Read the model definition and answer for the solid it produces. Units are mm, in the model's axes. A direction names the side the tool comes from. Give positions to 0.01 mm unless a question says otherwise; leave off trailing zeros. Loops run counter-clockwise (first coordinate to the right, second up) from the corner with the lowest first, then second, coordinate; pieces in that order, holes last. Notation, with made-up numbers: (49.5, -28) -> (79.5, -28) arc R23 cw to (79.5, -7) -> close; hole circle Ø3 at (63, 30). An arc over 180 degrees is marked (long way). Return JSON: item names as keys, results as strings. Group by question number.
from build123d import *

# Parameters (mm, degrees)
F0_W     = 76.2
F0_H     = 76.2
F1_DEPTH = 76.2
F2_W     = 58.42
F2_H     = 58.42
F3_DEPTH = 76.2
F4_W     = 58.42
F4_H     = 67.31
F5_DEPTH = 76.2
F6_W     = 58.42
F6_H     = 134.62
F7_DEPTH = 76.2


with BuildPart() as f1:
    # F0 (on Top) → F1 (new body)
    with BuildSketch(Plane.XY):
        with Locations((38.1, -38.1)):
            Rectangle(F0_W, F0_H)
    extrude(amount=F1_DEPTH)

    # F2 (on face) → F3 (cut)
    with BuildSketch(Plane.XY.offset(76.2)):
        with Locations((38.1, -38.1)):
            Rectangle(F2_W, F2_H)
    extrude(amount=-F3_DEPTH, mode=Mode.SUBTRACT)

    # F4 (on face) → F5 (cut)
    with BuildSketch(Plane.YZ.offset(76.2)):
        with Locations((-38.1, 33.655)):
            Rectangle(F4_W, F4_H)
    extrude(amount=-F5_DEPTH, mode=Mode.SUBTRACT)

    # F6 (on face) → F7 (cut)
    with BuildSketch(Plane.XZ.offset(76.2)):
        with Locations((38.1, 0)):
            Rectangle(F6_W, F6_H)
    extrude(amount=-F7_DEPTH, mode=Mode.SUBTRACT)


solid = f1.part
1. Which of the six approach directions +Z, -Z, +X, -X, +Y, -Y give full straight-line access (tool end or side, diameter ignored) to faces 5 (the flat face through (72, -39, 67.31)), 6 (the flat face through (38, -76.2, 69)), 7 (the flat face through (8.89, -72, 33)), 8 (the flat face through (4, -72, 0)), 9 (the flat face through (67.31, -39, 72))?
2. Section B-B on z = 33.5 is taken. Determine the outline of the cut face in (x, y), then the cut area to 3 significant figures.
3. A flat-ended cylindrical pin translates along its axis: pin 1 Ø4.5 at (x, y) = (72.5, -27.5) entering from -Z. Find the tip coordinate at first contact, or state that the pin passes through.
4. Section D-D on z = 71.5 is taken. Determine the outline of the cut face in (x, y).
5. Determine the mould class of faces 1 (the flat face through (72, -4, 0)), 2 (the flat face through (76.2, -38, 69)), 3 (the flat face through (39, -67.31, 72)), 4 (the flat face through (38, -5, 67.31)) for opening direction X: pulls with the +X half, pulls with the -X half, needs draft (parallel to the pull), parting line crosses it, or undercut.
6. Straight lines are drawn through the part: line 1 (Y direction, x = 70.5, z = 56); line 2 (X direction, y = -4.5, z = 48.5); line 3 (Z direction, x = 65, y = -2.5). For each, find the intervals that lie inside material, in ascending order. Write a range as from..to.
7. Section A-A on y = -14 is taken. Determine the outline of the cut face in (x, z).
8. Section C-C on x = 44 is taken. Determine the outline of the cut face in (y, z).
Completed:
{
 "1": {"face 5": "-Z, +X, -X", "face 6": "+Z, -Z, +X, -X, -Y", "face 7": "-Z, +Y, -Y", "face 8": "-Z, +X, -X, +Y, -Y", "face 9": "+Z, -Z"},
 "2": {"outline": "(0, -76.2) -> (8.89, -76.2) -> (8.89, -67.31) -> (0, -67.31) -> close; (0, -8.89) -> (8.89, -8.89) -> (8.89, 0) -> (0, 0) -> close; (67.31, -76.2) -> (76.2, -76.2) -> (76.2, -67.31) -> (67.31, -67.31) -> close; (67.31, -8.89) -> (76.2, -8.89) -> (76.2, 0) -> (67.31, 0) -> close", "area": "316 mm²"},
 "3": {"pin 1": "stops at z = 67.31"},
 "4": {"outline": "(0, -76.2) -> (76.2, -76.2) -> (76.2, 0) -> (0, 0) -> close; hole (8.89, -67.31) -> (67.31, -67.31) -> (67.31, -8.89) -> (8.89, -8.89) -> close"},
 "5": {"face 1": "needs draft", "face 2": "pulls with the +X half", "face 3": "undercut", "face 4": "undercut"},
 "6": {"line 1": "y = -76.2..-67.31, -8.89..0", "line 2": "x = 0..8.89, 67.31..76.2", "line 3": "z = 67.31..76.2"},
 "7": {"outline": "(0, 67.31) -> (8.89, 67.31) -> (8.89, 76.2) -> (0, 76.2) -> close; (67.31, 67.31) -> (76.2, 67.31) -> (76.2, 76.2) -> (67.31, 76.2) -> close"},
 "8": {"outline": "(-76.2, 67.31) -> (-67.31, 67.31) -> (-67.31, 76.2) -> (-76.2, 76.2) -> close; (-8.89, 67.31) -> (0, 67.31) -> (0, 76.2) -> (-8.89, 76.2) -> close"}
}
